Work out the finished part from the listing and answer in its coordinate system (mm). A direction names the side the tool comes from. Give positions to 0.01 mm unless a question says otherwise; leave off trailing zeros. Loops run counter-clockwise (first coordinate to the right, second up) from the corner with the lowest first, then second, coordinate; pieces in that order, holes last. Notation, with made-up numbers: (-24, 76.25) - (-7, 76.25) arc R29 cw to (-7, 99.25) - close; hole circle Ø5 at (68.25, 41). An arc over 180 degrees is marked (long way). One line per question, with ' | ' between items. Start each with the question number.
1. Find the intervals of material crossed by line 1 (Z direction, x = 0, y = 0); line 2 (Y direction, x = 0.25, z = 0); line 3 (Z direction, x = 0.75, y = -2), in increasing order.
2. Each of these flat-tipped pins is pushed along its axis until it touches: pin 1 (2 mm diameter, centred on x = 0.5, y = 1, fed in from -Z); pin 2 (6 mm diameter, centred on y = 0, z = 0, fed in from +X); pin 3 (3 mm diameter, centred on x = 1.5, y = 12.5, fed in from +Z); pin 4 (1.5 mm diameter, centred on x = 1.5, z = 10.5, fed in from -Y). Where does it stop, or does it pass through?
3. Which of the six approach directions +Z, -Z, +X, -X, +Y, -Y give full straight-line access (tool end or side, diameter ignored) to faces 4 (the face through (0.044, 27.292, 5.813)), 5 (the face through (0.044, -5.077, -0.175)), 6 (the face through (0.044, 27.362, -5.828))?
4. Section A-A (y = 0) is taken. Determine the outline of the cut face in (x, z) (3 decimals), plus the area to 3 significant figures.
5. Section D-D (y = 11) is taken. Determine the outline of the cut face in (x, z) (3 decimals).
6. Section B-B (z = 0) is taken. Determine the outline of the cut face in (x, y) (3 decimals), plus the area to 3 significant figures.
7. Section C-C (x = -2.5) is taken. Determine the outline of the cut face in (y, z) (3 decimals), plus the area to 3 significant figures.
8. For a pull along Z with two mould halves and no side action, classify faces 1 (the face through (0.04, 30.48, 0.09)), 2 (the face through (-3.175, 3, -5)), 3 (the face through (0, 3.966, 0)) as released by +Z, released by -Z, zero draft, split by the parting line, or undercut.
from build123d import *

# Parameters (mm, degrees)
SKETCH1_R           = 25.4
BOSS_EXTRUDE1_DEPTH = 3.175
BOSS_EXTRUDE2_DEPTH = 3.175


with BuildPart() as part:
    # Sketch1 → Boss-Extrude1 (new, symmetric)
    with BuildSketch(Plane(origin=(0, 0, 0), x_dir=(0, 0, -1), z_dir=(1, 0, 0))):
        Circle(SKETCH1_R)
        with BuildLine():
            Line((-3.175, 3.965573729), (3.175, 3.965573729))
            ThreePointArc((3.175, 3.965573729), (0, -5.08), (-3.175, 3.965573729))
        make_face(mode=Mode.SUBTRACT)
    extrude(amount=BOSS_EXTRUDE1_DEPTH, both=True)

    # Sketch2 → Boss-Extrude2 (add, symmetric)
    with BuildSketch(Plane(origin=(0, 0, 0), x_dir=(0, 0, -1), z_dir=(1, 0, 0))):
        with BuildLine():
            Line((-5.291666667, 24.842670225), (-6.35, 29.81120427))
            ThreePointArc((-6.35, 29.81120427), (0, 30.48), (6.35, 29.81120427))
            Line((6.35, 29.81120427), (5.291666667, 24.842670225))
            ThreePointArc((5.291666667, 24.842670225), (0, 25.4), (-5.291666667, 24.842670225))
        make_face()
    extrude(amount=BOSS_EXTRUDE2_DEPTH, both=True)


solid = part.part
Conclusion:
1) line 1: -25.4 to -5.08, 5.08 to 25.4 | line 2: -25.4 to -5.08, 3.97 to 30.48 | line 3: -25.32 to -4.67, 4.67 to 25.32
2) pin 1: z = -25.4 | pin 2: through | pin 3: z = 22.89 | pin 4: y = -23.45
3) face 4: +Z, +X, -X | face 5: +X, -X | face 6: -Z, +X, -X
4) outline: (-3.175, -25.4) - (3.175, -25.4) - (3.175, -5.08) - (-3.175, -5.08) - close; (-3.175, 5.08) - (3.175, 5.08) - (3.175, 25.4) - (-3.175, 25.4) - close | area: 258 mm²
5) outline: (-3.175, -22.895) - (3.175, -22.895) - (3.175, 22.895) - (-3.175, 22.895) - close
6) outline: (-3.175, -25.4) - (3.175, -25.4) - (3.175, -5.08) - (-3.175, -5.08) - close; (-3.175, 3.966) - (3.175, 3.966) - (3.175, 30.48) - (-3.175, 30.48) - close | area: 297 mm²
7) outline: (24.843, -5.292) - (29.811, -6.35) arc R30.48 ccw to (29.811, 6.35) - (24.843, 5.292) arc R25.4 ccw (long way) to start; hole (3.966, -3.175) - (3.966, 3.175) arc R5.08 ccw (long way) to start | area: 2,010 mm²
8) face 1: split by the parting line | face 2: zero draft | face 3: undercut
